from build123d import *

# Parameters (mm, degrees)
ESBO_O1_R                = 100
RESSALTO_EXTRUS_O1_DEPTH = 5
ESBO_O2_R                = 1.5
CORTE_EXTRUS_O1_DEPTH    = 142.509716981


with BuildPart() as part:
    # Esboço1 → Ressalto-extrusão1 (new body)
    with BuildSketch(Plane(origin=(0, 0, 0), x_dir=(1, 0, 0), z_dir=(0, 1, 0))):
        with Locations(Location((0, 0, 0), (0, 0, 270))):
            Circle(ESBO_O1_R)
    extrude(amount=RESSALTO_EXTRUS_O1_DEPTH)

    # Esboço2 → Corte-extrusão1 (cut, through all)
    with BuildSketch(Plane(origin=(0, 5, 0), x_dir=(1, 0, 0), z_dir=(0, 1, 0))):
        with Locations(Location((-93, 18.5, 0), (0, 0, 270))):
            Circle(ESBO_O2_R)
        with Locations(Location((-55, 18.5, 0), (0, 0, 270))):
            Circle(ESBO_O2_R)
        with Locations(Location((-55, -18.5, 0), (0, 0, 270))):
            Circle(ESBO_O2_R)
        with Locations(Location((-93, -18.5, 0), (0, 0, 270))):
            Circle(ESBO_O2_R)
        with Locations(Location((52, 18.75, 0), (0, 0, 270))):
            Circle(ESBO_O2_R)
        with Locations(Location((89.5, 18.75, 0), (0, 0, 270))):
            Circle(ESBO_O2_R)
        with Locations(Location((52, -18.75, 0), (0, 0, 270))):
            Circle(ESBO_O2_R)
        with Locations(Location((89.5, -18.75, 0), (0, 0, 270))):
            Circle(ESBO_O2_R)
        with Locations(Location((30.47853003, -89.790362552, 0), (0, 0, 270))):
            Circle(ESBO_O2_R)
        with Locations(Location((11.47853003, -56.881397208, 0), (0, 0, 270))):
            Circle(ESBO_O2_R)
        with Locations(Location((43.52146997, -38.381397208, 0), (0, 0, 270))):
            Circle(ESBO_O2_R)
        with Locations(Location((62.52146997, -71.290362552, 0), (0, 0, 270))):
            Circle(ESBO_O2_R)
        with Locations(Location((-42.237976321, 35.658320997, 0), (0, 0, 270))):
            Circle(ESBO_O2_R)
        with Locations(Location((-60.987976321, 68.134273639, 0), (0, 0, 270))):
            Circle(ESBO_O2_R)
        with Locations(Location((-9.762023679, 54.408320997, 0), (0, 0, 270))):
            Circle(ESBO_O2_R)
        with Locations(Location((-28.512023679, 86.884273639, 0), (0, 0, 270))):
            Circle(ESBO_O2_R)
        with Locations(Location((62.52146997, 71.290362552, 0), (0, 0, 270))):
            Circle(ESBO_O2_R)
        with Locations(Location((43.52146997, 38.381397208, 0), (0, 0, 270))):
            Circle(ESBO_O2_R)
        with Locations(Location((11.47853003, 56.881397208, 0), (0, 0, 270))):
            Circle(ESBO_O2_R)
        with Locations(Location((30.47853003, 89.790362552, 0), (0, 0, 270))):
            Circle(ESBO_O2_R)
        with Locations(Location((-9.762023679, -54.408320997, 0), (0, 0, 270))):
            Circle(ESBO_O2_R)
        with Locations(Location((-28.512023679, -86.884273639, 0), (0, 0, 270))):
            Circle(ESBO_O2_R)
        with Locations(Location((-42.237976321, -35.658320997, 0), (0, 0, 270))):
            Circle(ESBO_O2_R)
        with Locations(Location((-60.987976321, -68.134273639, 0), (0, 0, 270))):
            Circle(ESBO_O2_R)
        Polygon((-37.5, 0), (-37.5, 8), (-44.5, 8), (-44.5, -8), (-37.5, -8), align=None)
        Polygon((18.75, -32.475952642), (11.82179677, -36.475952642), (15.32179677, -42.538130468), (29.17820323, -34.538130468), (25.67820323, -28.475952642), align=None)
        Polygon((18.75, 32.475952642), (25.67820323, 28.475952642), (29.17820323, 34.538130468), (15.32179677, 42.538130468), (11.82179677, 36.475952642), align=None)
    extrude(amount=-CORTE_EXTRUS_O1_DEPTH, mode=Mode.SUBTRACT)


solid = part.part
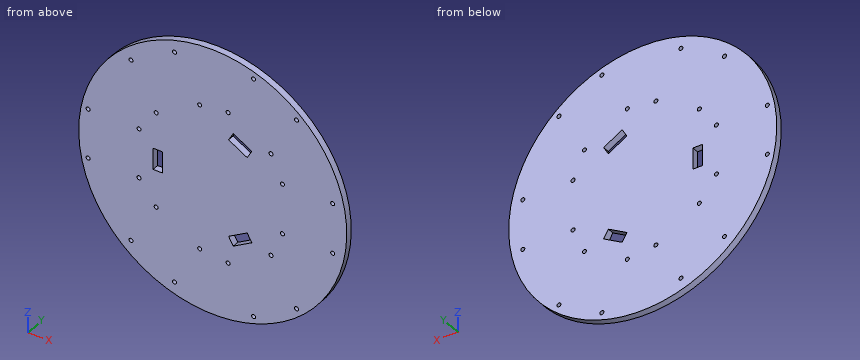
Build history of the part. All positions in model axes, mm. Coordinates: 2 decimals unless noted, no trailing zeros. Order: outer loops, then holes, each group sorted by start corner. A loop starts at its lowest first (then second) coordinate and runs counter-clockwise, first axis right, second up. Notation, with made-up numbers: (20.5, 65.25) -> (38.5, 65.25) arc R29 ccw to (38.5, 103.25) -> close; hole circle Ø5 at (4, 46). An arc over 180 degrees is marked (long way). One line per item, written item: value.
(1) Probe line 1 (Z direction, x = 89.5, y = 1.9); line 2 (Z direction, x = 16, y = 1.5); line 3 (X direction, y = 3.65, z = 36.5). List the from-to ranges inside material, lowest first. Write a range as [from, to].
Checked values:
line 1: [-44.61, -20.25], [-17.25, 17.25], [20.25, 44.61]
line 2: [-98.71, -42.15], [-34.06, 34.06], [42.15, 98.71]
line 3: [-93.1, -43.48], [-41, 11.84], [25.78, 93.1]
(2) Slice it at B-B, the plane z = -80. List the corners of the cut face in (x, y), plus the area to 3 significant figures.
Checked values:
outline: (-60, 0) -> (60, 0) -> (60, 5) -> (-60, 5) -> close
area: 600 mm2
(3) Drop flat-ended pins along their axis: pin 1 Ø1.5 at (y, z) = (1, -65.5) entering from -X; pin 2 Ø3 at (x, y) = (15.5, 1) entering from -Z; pin 3 Ø1.5 at (y, z) = (2, -3.5) entering from -X. Give the stop position or say it passes through.
Checked values:
pin 1: x = -76.21
pin 2: z = -99.02
pin 3: x = -99.96
(4) Slice it at A-A, the plane z = 0. List the corners of the cut face in (x, y), plus the area to 3 significant figures.
Checked values:
outline: (-100, 0) -> (-44.5, 0) -> (-44.5, 5) -> (-100, 5) -> close; (-37.5, 0) -> (100, 0) -> (100, 5) -> (-37.5, 5) -> close
area: 965 mm2
(5) Slice it at C-C, the plane y = 3.75. Count the separate pieces of the cut face and the enclosed holes in it, plus the area to 3 significant figures.
Checked values:
separate pieces: 1
enclosed holes: 27
area: 30,900 mm2
(6) Slice it at D-D, the plane x = 79. List the corners of the cut face in (y, z), plus the area to 3 significant figures.
Checked values:
outline: (0, -61.31) -> (5, -61.31) -> (5, 61.31) -> (0, 61.31) -> close
area: 613 mm2
